Input: dimensioned drawing with shaded views. Units: mm. Origin: part minimum x, y, z. Round coordinates to 2 decimals unless told otherwise and drop trailing zeros. Loops run counter-clockwise (first coordinate to the right, second up) from the corner with the lowest first, then second, coordinate; pieces in that order, holes last. Notation, with made-up numbers: M 26.25,7 L 69.25,7 A8 cw 69.25,14 Z; hole C 16.25,-22 d8. An arc over 180 degrees is marked long. Answer as a JSON object with one key per item and string values.
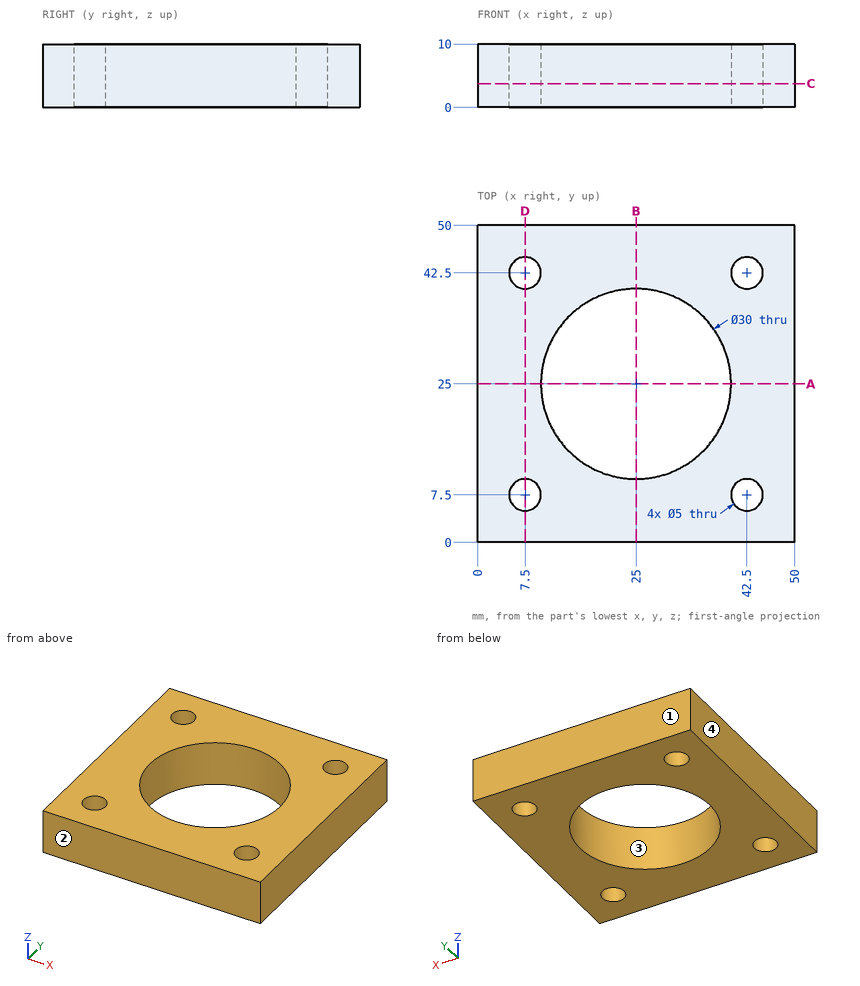
Item 1: Line query: probe 1 along Y at (x, z) = (7.5, 4.75); probe 2 along X at (y, z) = (41, 4.25); probe 3 along X at (y, z) = (40.5, 2). Output: solid intervals per line, ascending. Write a range as from..to.
Answer sheet:
{"probe 1": "y = 0..5, 10..40, 45..50", "probe 2": "x = 0..5.5, 9.5..40.5, 44.5..50", "probe 3": "x = 0..6, 9..41, 44..50"}
Item 2: Contact query for a flat-ended pin moving along its axis: pin 1 Ø4 at (x, y) = (7.5, 7.5) entering from +Z (3 decimals). Output: stop coordinate, or through.
Answer sheet:
{"pin 1": "passes through"}
Item 3: Section C-C on z = 3.75. Return the cut outline in (x, y).
Answer sheet:
{"outline": "M 0,0 L 50,0 L 50,50 L 0,50 Z; hole C 7.5,7.5 d5; hole C 7.5,42.5 d5; hole C 25,25 d30; hole C 42.5,7.5 d5; hole C 42.5,42.5 d5"}
Item 4: Pull-direction query (Y, two-part tool) for the marked faces 1, 2, 3 and 4; classes: pulls with the +Y half, pulls with the -Y half, needs draft (parallel to the pull), parting line crosses it, or undercut.
Answer sheet:
{"face 1": "pulls with the +Y half", "face 2": "pulls with the -Y half", "face 3": "undercut", "face 4": "needs draft"}
Item 5: Section A-A on y = 25. Return the cut outline in (x, z).
Answer sheet:
{"outline": "M 0,0 L 10,0 L 10,10 L 0,10 Z; M 40,0 L 50,0 L 50,10 L 40,10 Z"}
Item 6: Section D-D on x = 7.5. Return the cut outline in (y, z), then the cut area to 3 significant figures.
Answer sheet:
{"outline": "M 0,0 L 5,0 L 5,10 L 0,10 Z; M 10,0 L 40,0 L 40,10 L 10,10 Z; M 45,0 L 50,0 L 50,10 L 45,10 Z", "area": "400 mm²"}
